Here's the drawing with two shaded views (mm, measured from the low corner). I have some questions. A direction names the side the tool comes from. Round coordinates to 2 decimals unless told otherwise and drop trailing zeros.
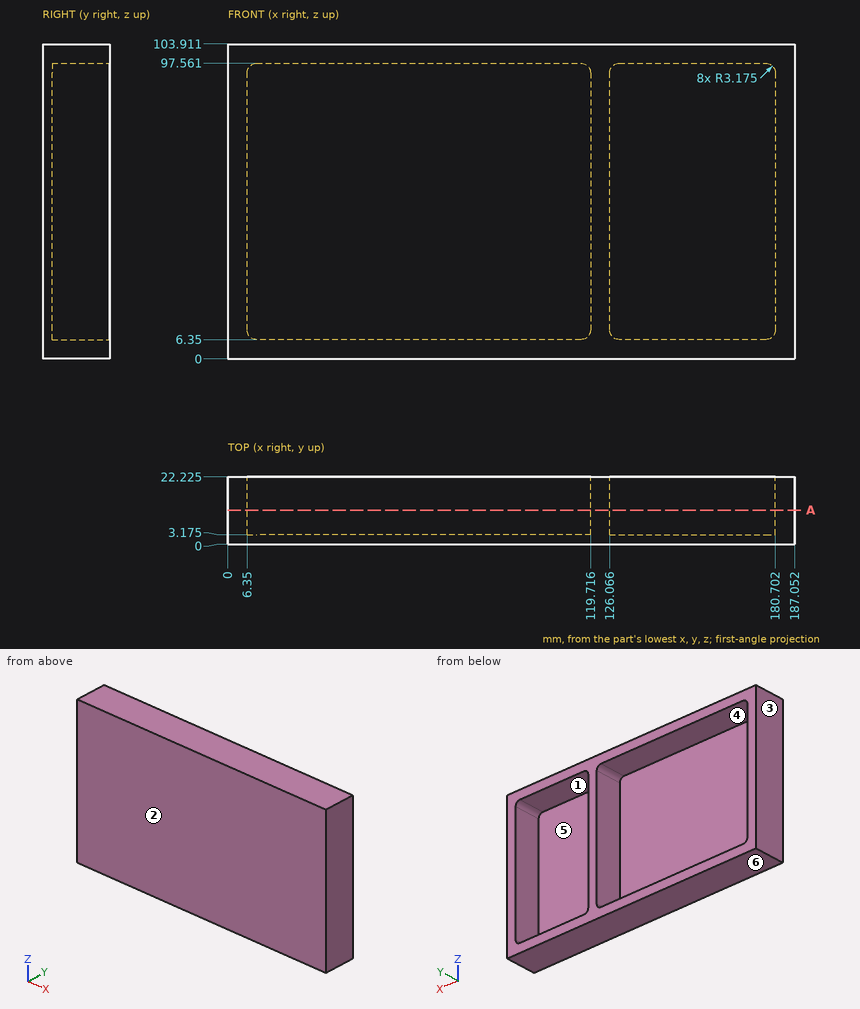
Q1. On a 3-axis mill with a long thin cutter (end or side, diameter ignored), from which of +Z, -Z, +X, -X, +Y, -Y can I reach the whole of each face in a straight line? I mean the marked faces 5 and 6. Say none if no direction works.
Q2. I'm going to push a flat-ended pin straight in: pin 1 Ø16.5 at (x, z) = (160, 30.5) entering from +Y (1 decimal). Where does the tip first touch, or does it pass through?
Q3. We'd pull the mould along X, two halves only. Please class the marked faces 1, 2, 3 and 4: pulls with the +X half, pulls with the -X half, needs draft (parallel to the pull), parting line crosses it, or undercut.
Q4. Imagine slicing it at A-A, the plane y = 11.25. Count the separate pieces of the cut face and the enclosed holes in it, then the cut area to 3 significant figures.
Q5. If I drill on L1, parallel to X at y = 15, z = 17.5; L2, parallel to Z at x = 81, y = 7.5; L3, parallel to Z at x = 117, y = 10.25, over which ranges is the centre line in solid material (lowest first)?
Results found:
1. face 5: +Y
1. face 6: -Z, +X, -X, +Y, -Y
2. pin 1: stops at y = 3.2
3. face 1: undercut
3. face 2: needs draft
3. face 3: pulls with the -X half
3. face 4: undercut
4. separate pieces: 1
4. enclosed holes: 2
4. area: 4,130 mm2
5. L1: x = 0 to 6.35, 119.72 to 126.07, 180.7 to 187.05
5. L2: z = 0 to 6.35, 97.56 to 103.91
5. L3: z = 0 to 6.38, 97.53 to 103.91
